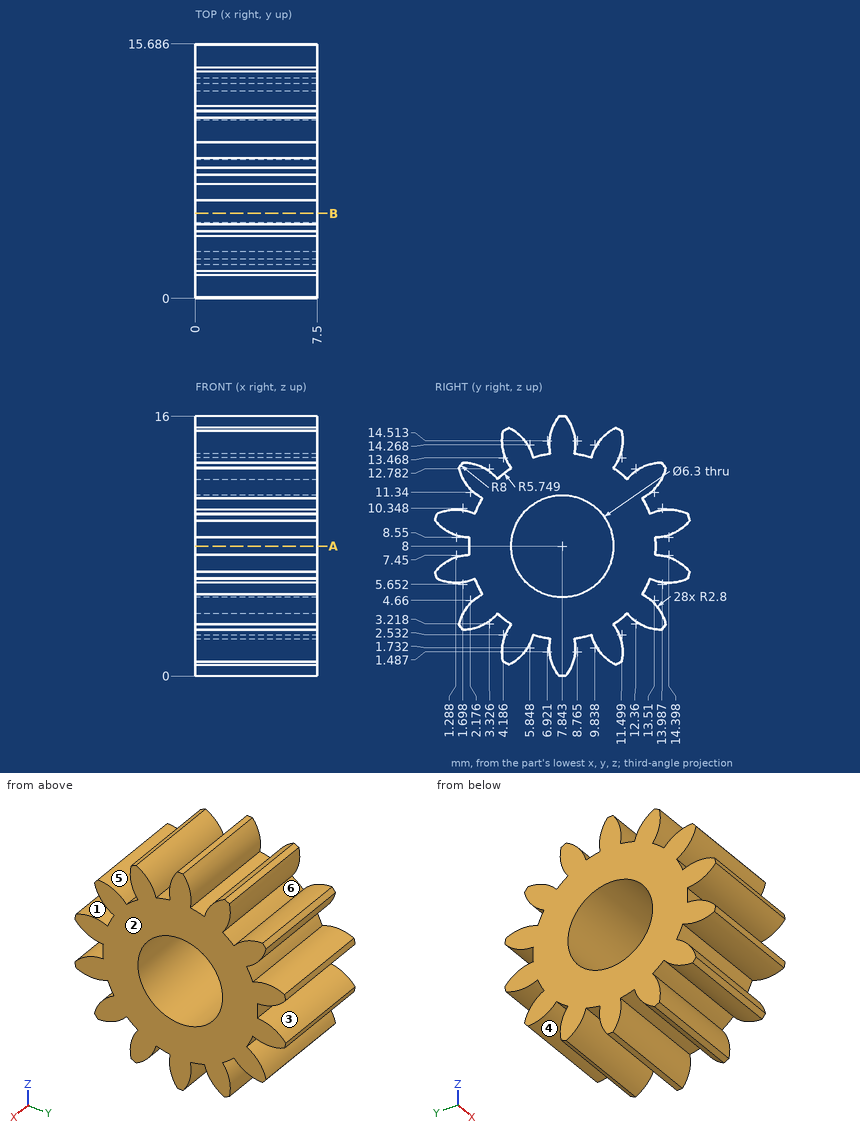
Verification items for this drawing (mm, ordinates from the low corner). A direction names the side the tool comes from. Round coordinates to 2 decimals unless told otherwise and drop trailing zeros. Order: outer loops, then holes, each group sorted by start corner. A loop starts at its lowest first (then second) coordinate and runs counter-clockwise, first axis right, second up. Notation, with made-up numbers: M 16.25,7 L 52.25,7 A20 ccw 52.25,17 Z; hole C -23.5,-7.5 d9. An arc over 180 degrees is marked long. Answer in a Markdown table with one row per item. Add a question column.
Item 1: Material ranges on L1, parallel to Z at x = 3.75, y = 8; L2, parallel to Y at x = 5.25, z = 8; L3, parallel to Z at x = 7.25, y = 9, recorded low to high. Write a range as [from, to].
Item 2: Sectioned sample at A-A, the plane z = 8. Enter the section's corners in (x, y).
Item 3: Sectioned sample at B-B, the plane y = 5.25. Enter the section's corners in (x, z) (1 decimal).
Item 4: Set-up check for the marked faces 4, 5 and 6: record each of +Z, -Z, +X, -X, +Y, -Y from which the full face is reachable in a straight line by a thin tool's end or side.
Item 5: Depth check by flat-ended pin: pin 1 Ø2 at (x, y) = (3.5, 3.5) entering from -Z. Enter the tip coordinate at first touch or a pass-through.
Item 6: Draft check along Y on the marked faces 1, 2 and 3. Enter one of: released by +Y, released by -Y, zero draft, split by the parting line, or undercut.
Filled in:
| question | item | result |
|---|---|---|
| 1 | L1 | z = [0, 4.85], [11.15, 16] |
| 1 | L2 | y = [2.09, 4.69], [10.99, 13.59] |
| 1 | L3 | z = [2.37, 5.07], [10.93, 13.63] |
| 2 | outline | M 0,2.09 L 7.5,2.09 L 7.5,4.69 L 0,4.69 Z; M 0,10.99 L 7.5,10.99 L 7.5,13.59 L 0,13.59 Z |
| 3 | outline | M 0,1.2 L 7.5,1.2 L 7.5,6.2 L 0,6.2 Z; M 0,9.8 L 7.5,9.8 L 7.5,14.8 L 0,14.8 Z |
| 4 | face 4 | -Z, +X, -X |
| 4 | face 5 | +Z, +X, -X |
| 4 | face 6 | +X, -X |
| 5 | pin 1 | stops at z = 0.73 |
| 6 | face 1 | undercut |
| 6 | face 2 | zero draft |
| 6 | face 3 | released by +Y |
